Could you check a few things on this model? Use its own coordinates, in mm. A direction names the side the tool comes from. Give positions to 0.01 mm unless a question says otherwise; leave off trailing zeros. Write each loop counter-clockwise with the first axis right and the second up, starting at its lowest first coordinate (ties: lowest second). Pieces come first, ordered by that corner, then holes. Notation, with made-up numbers: M -22,87.25 L -11,87.25 A19 cw -11,113.25 Z; hole C 38,64 d10. An arc over 180 degrees is marked long. One line per item, written item: value.
```python
from build123d import *

# Parameters (mm, degrees)
SKETCH1_W           = 90
SKETCH1_H           = 177
BOSS_EXTRUDE1_DEPTH = 1.6
BOSS_EXTRUDE4_DEPTH = 1.6
BOSS_EXTRUDE5_DEPTH = 1.6
SKETCH9_W           = 70.7486
SKETCH9_H           = 57
CUT_EXTRUDE3_DEPTH  = 2.6
FILLET1_R           = 3


with BuildPart() as part:
    # Sketch1 → Boss-Extrude1 (new body)
    with BuildSketch(Plane(origin=(0, 0, 0), x_dir=(1, 0, 0), z_dir=(0, 1, 0))):
        Rectangle(SKETCH1_W, SKETCH1_H)
    extrude(amount=BOSS_EXTRUDE1_DEPTH)

    # Sketch7 → Boss-Extrude4 (add)
    with BuildSketch(Plane.XZ):
        Polygon((-45, -88.5), (-45, -30.1257), (-48.3743, -33.5), (-48.3743, -88.5), align=None)
        Polygon((45, -30.1257), (45, -88.5), (48.3743, -88.5), (48.3743, -33.5), align=None)
    extrude(amount=-BOSS_EXTRUDE4_DEPTH)

    # Sketch w → Boss-Extrude5 (add)
    with BuildSketch(Plane(origin=(0, 1.6, 0), x_dir=(1, 0, 0), z_dir=(0, 1, 0))):
        Polygon((-43, -90.5), (43, -90.5), (45, -88.5), (-45, -88.5), align=None)
        Polygon((45, -35.5), (45, -88.5), (49, -84.5), (49, -39.5), align=None)
        Polygon((45, 19.5), (45, -30.5), (49, -26.5), (49, 15.5), align=None)
    extrude(amount=-BOSS_EXTRUDE5_DEPTH)

    # Sketch9 → Cut-Extrude3 (cut, through all)
    with BuildSketch(Plane.XZ):
        with Locations((0, -60)):
            Rectangle(SKETCH9_W, SKETCH9_H)
    extrude(amount=-CUT_EXTRUDE3_DEPTH, mode=Mode.SUBTRACT)

    # Fillet1
    fillet1_edges = [part.edges().sort_by_distance(p)[0] for p in [
        (-45, 0.8, -30.1257),
        (45, 0.8, -30.1257),
        (45, 0.8, 35.5),
        (45, 0.8, 30.5),
        (45, 0.8, -19.5),
        (-35.3743, 0.8, -31.5),
        (35.3743, 0.8, -31.5),
    ]]
    fillet(fillet1_edges, radius=FILLET1_R)


solid = part.part
```
1) If we section it at B-B, the plane y = 0.75: Write out the boundary of the cut face in (x, z).
Outcome:
outline: M -48.37,-88.5 L -35.37,-88.5 L -35.37,-34.5 A3 cw -32.37,-31.5 L 32.37,-31.5 A3 cw 35.37,-34.5 L 35.37,-88.5 L 48.37,-88.5 L 48.37,-33.5 L 45.88,-31 A3 cw 45,-28.88 L 45,-20.74 A3 cw 45.88,-18.62 L 49,-15.5 L 49,26.5 L 45.88,29.62 A3 cw 45,31.74 L 45,34.26 A3 cw 45.88,36.38 L 49,39.5 L 49,84.5 L 43,90.5 L -43,90.5 L -45,88.5 L -45,-28.88 A3 cw -45.88,-31 L -48.37,-33.5 Z
2) Please list where these lines run through material, in increasing order: L1, parallel to X at y = 1, z = -68.5; L2, parallel to Z at x = -20.5, y = 0.15; L3, parallel to X at y = 1.5, z = 10.5. Write a range as from..to.
Outcome:
L1: x = -48.37..-35.37, 35.37..48.37
L2: z = -31.5..90.5
L3: x = -45..49
3) If we section it at A-A, the plane z = -50: Write out the boundary of the cut face in (x, y).
Outcome:
outline: M -48.37,0 L -35.37,0 L -35.37,1.6 L -48.37,1.6 Z; M 35.37,0 L 48.37,0 L 48.37,1.6 L 35.37,1.6 Z
4) We'd pull the mould along Z, two halves only. Please class faces 3 (the face through (0, 0, 20)), 4 (the face through (46, 0.8, 87.5)), 5 (the face through (47.4, 0.8, 28.1)): pulls with the +Z half, pulls with the -Z half, needs draft (parallel to the pull), parting line crosses it, or undercut.
Outcome:
face 3: needs draft
face 4: pulls with the +Z half
face 5: undercut
5) If we section it at C-C, the plane x = 22: Write out the boundary of the cut face in (y, z).
Outcome:
outline: M 0,-31.5 L 1.6,-31.5 L 1.6,90.5 L 0,90.5 Z
6) If we section it at D-D, the plane z = 3.5: Write out the boundary of the cut face in (x, y).
Outcome:
outline: M -45,0 L 49,0 L 49,1.6 L -45,1.6 Z
7) I'm going to push flat-ended pins straight in: pin 1 (0.8 mm diameter, centred on y = 1, z = -54.5, fed in from +X); pin 2 (0.5 mm diameter, centred on y = 1, z = 33.5, fed in from +X); pin 3 (0.8 mm diameter, centred on x = -12.5, y = 0.5, fed in from -Z). Where does each tip first touch, or does it pass through?
Outcome:
pin 1: stops at x = 48.37
pin 2: stops at x = 45
pin 3: stops at z = -31.5
8) On a 3-axis mill with a long thin cutter (end or side, diameter ignored), from which of +Z, -Z, +X, -X, +Y, -Y can I reach the whole of each face in a straight line? I mean faces 1 (the face through (0, 1.6, 20)), 2 (the face through (47.5, 0.8, -17)). Say none if no direction works.
Outcome:
face 1: +Z, -Z, +X, -X, +Y
face 2: +X, +Y, -Y
